from build123d import *

# Parameters (mm, degrees)
SKETCH1_R           = 12.7
BOSS_EXTRUDE1_DEPTH = 50.8
FILLET1_R           = 2.54
FILLET2_R           = 2.54


with BuildPart() as part:
    # Sketch1 → Boss-Extrude1 (new body)
    with BuildSketch(Plane(origin=(0, 0, 0), x_dir=(0, 0, -1), z_dir=(1, 0, 0))):
        with BuildLine():
            Line((-95.25, 0), (0, 0))
            Line((0, 0), (0, 70.939487758))
            ThreePointArc((0, 70.939487758), (-6.35, 69.85), (-12.7, 70.939487758))
            Line((-12.7, 70.939487758), (-12.7, 6.35))
            Line((-12.7, 6.35), (-95.25, 6.35))
            Line((-95.25, 6.35), (-95.25, 0))
        make_face()
        with BuildLine():
            Line((-12.7, 70.939487758), (0, 70.939487758))
            ThreePointArc((0, 70.939487758), (9.204259867, 77.901477372), (12.7, 88.9))
            ThreePointArc((12.7, 88.9), (-17.348522628, 104.454259867), (-12.7, 70.939487758))
        make_face()
        with Locations((-6.35, 88.9)):
            Circle(SKETCH1_R, mode=Mode.SUBTRACT)
        with BuildLine():
            ThreePointArc((-12.7, 70.939487758), (-6.35, 69.85), (0, 70.939487758))
            Line((0, 70.939487758), (-12.7, 70.939487758))
        make_face()
    extrude(amount=BOSS_EXTRUDE1_DEPTH)

    # Fillet1
    fillet1_edges = [part.edges().sort_by_distance(p)[0] for p in [
        (25.4, 6.35, 12.7),
        (25.4, 70.939487758, 12.7),
        (25.4, 70.939487758, 0),
    ]]
    fillet(fillet1_edges, radius=FILLET1_R)

    # Fillet2
    fillet2_edges = [part.edges().sort_by_distance(p)[0] for p in [
        (25.4, 6.35, 95.25),
    ]]
    fillet(fillet2_edges, radius=FILLET2_R)


solid = part.part
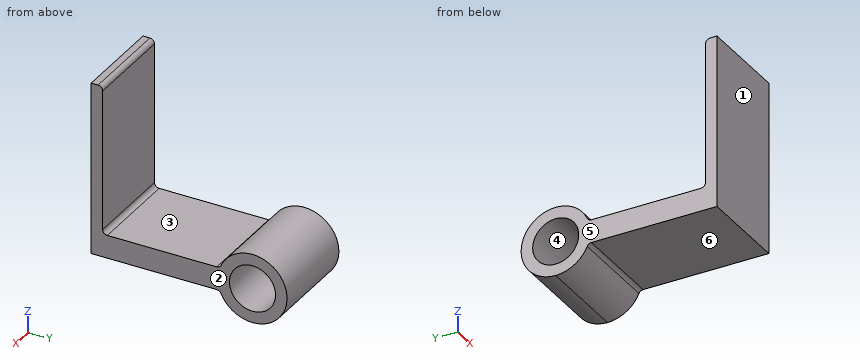
Design review of the part built by this model. Coordinates are the model's own, in mm. Face numbers are marked on the shaded views. A direction names the side the tool comes from. Give positions to 0.01 mm unless a question says otherwise; leave off trailing zeros. Order: outer loops, then holes, each group sorted by start corner. A loop starts at its lowest first (then second) coordinate and runs counter-clockwise, first axis right, second up.
1. Add section B-B, the plane x = 40. State the section outline as (y, z) points.
Solution:
outline: (0, 0) - (69.23, 0) arc R2.54 cw to (71.54, -1.49) arc R19.05 ccw (long way) to (71.54, 14.19) arc R2.54 cw to (69.23, 12.7) - (8.89, 12.7) arc R2.54 cw to (6.35, 15.24) - (6.35, 92.71) arc R2.54 ccw to (3.81, 95.25) - (0, 95.25) - close; hole circle Ø25.4 at (88.9, 6.35)
2. Mouldability with a two-part tool opening along Y and no side actions: class the marked faces 1, 2, 3 and 4 as +Y half, -Y half, draft (parallel to the pull), parting line (faces both ways), or undercut.
Solution:
face 1: -Y half
face 2: draft
face 3: undercut
face 4: undercut
3. Add section A-A, the plane z = 6.35. State the section outline as (x, y) points, then the cut area to 3 significant figures.
Solution:
outline: (0, 0) - (50.8, 0) - (50.8, 76.2) - (0, 76.2) - close; (0, 101.6) - (50.8, 101.6) - (50.8, 107.95) - (0, 107.95) - close
area: 4,190 mm2
4. To check wall thickness, follow L1, parallel to Y at x = 37, z = 6; L2, parallel to Z at x = 43.5, y = 89; L3, parallel to Y at x = 8, z = 15.5. State the ranges of each line that lie inside material, in increasing order.
Solution:
L1: y = 0 to 76.2, 101.6 to 107.95
L2: z = -12.7 to -6.35, 19.05 to 25.4
L3: y = 0 to 6.35, 72.19 to 80.09, 97.71 to 105.61
5. For pin 1 Ø8 at (x, y) = (21, 82) entering from -Z; pin 2 Ø4 at (x, y) = (39.5, 22.5) entering from -Z; pin 3 Ø2 at (x, y) = (40.5, 91.5) entering from -Z; pin 4 Ø8 at (y, z) = (93.5, 3) entering from -X, all flat-tipped, find the tip position at first contact; note any pin that passes through.
Solution:
pin 1: stops at z = -12.48
pin 2: stops at z = 0
pin 3: stops at z = -12.63
pin 4: passes through
6. Tool access review of the marked faces 5 and 6: name each direction out of +Z, -Z, +X, -X, +Y, -Y from which nothing blocks a thin tool from reaching the whole face with its end or side.
Solution:
face 5: +Z, -Z, -X, +Y, -Y
face 6: -Z, +X, -X, -Y
7. Add section D-D, the plane z = 76. State the section outline as (x, y) points.
Solution:
outline: (0, 0) - (50.8, 0) - (50.8, 6.35) - (0, 6.35) - close
8. Add section C-C, the plane y = 60. State the section outline as (x, z) points, then the cut area to 3 significant figures.
Solution:
outline: (0, 0) - (50.8, 0) - (50.8, 12.7) - (0, 12.7) - close
area: 645 mm2
